```python
from build123d import *

# Parameters (mm, degrees)
ESQUISSE1_W        = 80
ESQUISSE1_H        = 40
ESQUISSE1_R        = 7.5
ESQUISSE1_R_2      = 2.069624396
BOSS_EXTRU_1_DEPTH = 5


with BuildPart() as part:
    # Esquisse1 → Boss.-Extru.1 (new body)
    # profile 1 of 13: a face of its own
    with BuildSketch(Plane.XY):
        with Locations((0, -3.377163011)):
            Rectangle(ESQUISSE1_W, ESQUISSE1_H)
        with Locations((0, -3.377163011)):
            Circle(ESQUISSE1_R, mode=Mode.SUBTRACT)
        with Locations((32, -15.377163011)):
            Circle(ESQUISSE1_R_2, mode=Mode.SUBTRACT)
        with Locations((-32, 8.622836989)):
            Circle(ESQUISSE1_R_2, mode=Mode.SUBTRACT)
        with Locations((32, 8.622836989)):
            Circle(ESQUISSE1_R_2, mode=Mode.SUBTRACT)
        with Locations((-32, -15.377163011)):
            Circle(ESQUISSE1_R_2, mode=Mode.SUBTRACT)
    # profile 2 of 13: a face of its own
    with BuildSketch(Plane.XY):
        with BuildLine():
            ThreePointArc((-34.062905963, 8.789462695), (-33.792347303, 7.588024791), (-32.887150887, 6.752995165))
            ThreePointArc((-32.887150887, 6.752995165), (-33.267182328, 7.89122893), (-34.062905963, 8.789462695))
        make_face()
    # profile 3 of 13: a face of its own
    with BuildSketch(Plane.XY):
        with BuildLine():
            ThreePointArc((-33.175755077, 10.326053105), (-32, 10.086053105), (-30.824244923, 10.326053105))
            ThreePointArc((-30.824244923, 10.326053105), (-32, 10.692461384), (-33.175755077, 10.326053105))
        make_face()
    # profile 4 of 13: a face of its own
    with BuildSketch(Plane.XY):
        with BuildLine():
            ThreePointArc((-31.112849113, 6.752995165), (-30.250798145, 7.516655263), (-29.930375604, 8.622836989))
            ThreePointArc((-29.930375604, 8.622836989), (-29.932055895, 8.706217537), (-29.937094037, 8.789462695))
            ThreePointArc((-29.937094037, 8.789462695), (-30.732817672, 7.89122893), (-31.112849113, 6.752995165))
        make_face()
    # profile 5 of 13: a face of its own
    with BuildSketch(Plane.XY):
        with BuildLine():
            ThreePointArc((-29.930375604, -15.377163011), (-30.250798145, -14.270981286), (-31.112849113, -13.507321188))
            ThreePointArc((-31.112849113, -13.507321188), (-30.732817672, -14.645554953), (-29.937094037, -15.543788718))
            ThreePointArc((-29.937094037, -15.543788718), (-29.932055895, -15.46054356), (-29.930375604, -15.377163011))
        make_face()
    # profile 6 of 13: a face of its own
    with BuildSketch(Plane.XY):
        with BuildLine():
            ThreePointArc((-34.062905963, -15.543788718), (-33.267182328, -14.645554953), (-32.887150887, -13.507321188))
            ThreePointArc((-32.887150887, -13.507321188), (-33.792347303, -14.342350814), (-34.062905963, -15.543788718))
        make_face()
    # profile 7 of 13: a face of its own
    with BuildSketch(Plane.XY):
        with BuildLine():
            ThreePointArc((-30.824244923, -17.080379128), (-32, -16.840379128), (-33.175755077, -17.080379128))
            ThreePointArc((-33.175755077, -17.080379128), (-32, -17.446787407), (-30.824244923, -17.080379128))
        make_face()
    # profile 8 of 13: a face of its own
    with BuildSketch(Plane.XY):
        with BuildLine():
            ThreePointArc((30.824244923, 10.326053105), (32, 10.086053105), (33.175755077, 10.326053105))
            ThreePointArc((33.175755077, 10.326053105), (32, 10.692461384), (30.824244923, 10.326053105))
        make_face()
    # profile 9 of 13: a face of its own
    with BuildSketch(Plane.XY):
        with BuildLine():
            ThreePointArc((29.937094037, 8.789462695), (30.207652697, 7.588024791), (31.112849113, 6.752995165))
            ThreePointArc((31.112849113, 6.752995165), (30.732817672, 7.89122893), (29.937094037, 8.789462695))
        make_face()
    # profile 10 of 13: a face of its own
    with BuildSketch(Plane.XY):
        with BuildLine():
            ThreePointArc((34.062905963, 8.789462695), (33.267182328, 7.89122893), (32.887150887, 6.752995165))
            ThreePointArc((32.887150887, 6.752995165), (33.749201855, 7.516655263), (34.069624396, 8.622836989))
            ThreePointArc((34.069624396, 8.622836989), (34.067944105, 8.706217537), (34.062905963, 8.789462695))
        make_face()
    # profile 11 of 13: a face of its own
    with BuildSketch(Plane.XY):
        with BuildLine():
            ThreePointArc((34.062905963, -15.543788718), (34.067944105, -15.46054356), (34.069624396, -15.377163011))
            ThreePointArc((34.069624396, -15.377163011), (33.749201855, -14.270981286), (32.887150887, -13.507321188))
            ThreePointArc((32.887150887, -13.507321188), (33.267182328, -14.645554953), (34.062905963, -15.543788718))
        make_face()
    # profile 12 of 13: a face of its own
    with BuildSketch(Plane.XY):
        with BuildLine():
            ThreePointArc((29.937094037, -15.543788718), (30.732817672, -14.645554953), (31.112849113, -13.507321188))
            ThreePointArc((31.112849113, -13.507321188), (30.207652697, -14.342350814), (29.937094037, -15.543788718))
        make_face()
    # profile 13 of 13: a face of its own
    with BuildSketch(Plane.XY):
        with BuildLine():
            ThreePointArc((30.824244923, -17.080379128), (32, -17.446787407), (33.175755077, -17.080379128))
            ThreePointArc((33.175755077, -17.080379128), (32, -16.840379128), (30.824244923, -17.080379128))
        make_face()
    extrude(amount=BOSS_EXTRU_1_DEPTH)


solid = part.part
```
Geometry: final body of the model. Coordinates: model frame, mm. A direction names the side the tool comes from. Coordinates: 2 decimals unless noted, no trailing zeros. Order: outer loops, then holes, each group sorted by start corner. A loop starts at its lowest first (then second) coordinate and runs counter-clockwise, first axis right, second up. Notation, with made-up numbers: (-19.75, -16.75) -> (12.25, -16.75) arc R22 ccw to (12.25, 5.25) -> close; hole circle Ø1 at (58.5, 5). An arc over 180 degrees is marked (long way). Write each question's results on one line, items separated by ' | '. Start each with the question number.
1) Cut plane C-C, the plane z = 2.1. State how many separate pieces and enclosed holes the cut face has, and give its area (3 significant figures).
2) Cut plane D-D, the plane y = 7.5. Output: boundary loops of the cut face in (x, z), and give its area (3 significant figures).
3) First-contact query: pin 1 (12 mm diameter, centred on x = 25.5, y = -10.5, fed in from -Z). Flat tip, straight axial feed; report the tip coordinate or a pass-through.
4) Cut plane B-B, the plane y = 1.5. Output: boundary loops of the cut face in (x, z), and give its area (3 significant figures).
5) Material intervals for line 1 along Y through (x, z) = (0, 3.9); line 2 along X through (y, z) = (-16, 3.45); line 3 along Y through (x, z) = (30.5, 1.2), sorted ascending.
6) Set-up query: faces 1 (the flat face through (-1, 16.623, 2)), 2 (the cylindrical face through (-33.786, 9.669, 2.465)). Return all of +Z, -Z, +X, -X, +Y, -Y with unobstructed straight access to the full face (end or side cutting, diameter ignored); none if empty.
7) Cut plane A-A, the plane x = 0. Output: boundary loops of the cut face in (y, z).
8) Mould query, pull axis X, two halves, no side actions, for faces 3 (the cylindrical face through (-32.013, 6.553, 2.465)), 4 (the flat face through (40, -4, 2)), 5 (the flat face through (-1, 6, 0)). Classes: released by +X, released by -X, zero draft, split by the parting line, or undercut.
Checks:
1) separate pieces: 1 | enclosed holes: 5 | area: 2,980 mm^2
2) outline: (-40, 0) -> (-33.08, 0) -> (-33.08, 5) -> (-40, 5) -> close; (-30.92, 0) -> (30.92, 0) -> (30.92, 5) -> (-30.92, 5) -> close; (33.08, 0) -> (40, 0) -> (40, 5) -> (33.08, 5) -> close | area: 378 mm^2
3) pin 1: z = 0
4) outline: (-40, 0) -> (-5.7, 0) -> (-5.7, 5) -> (-40, 5) -> close; (5.7, 0) -> (40, 0) -> (40, 5) -> (5.7, 5) -> close | area: 343 mm^2
5) line 1: -23.38 to -10.88, 4.12 to 16.62 | line 2: -40 to -33.97, -30.03 to 30.03, 33.97 to 40 | line 3: -23.38 to -16.8, -14.99 to 8.24, 10.05 to 16.62
6) face 1: +Z, -Z, +X, -X, +Y | face 2: +Z, -Z
7) outline: (-23.38, 0) -> (-10.88, 0) -> (-10.88, 5) -> (-23.38, 5) -> close; (4.12, 0) -> (16.62, 0) -> (16.62, 5) -> (4.12, 5) -> close
8) face 3: undercut | face 4: released by +X | face 5: zero draft
